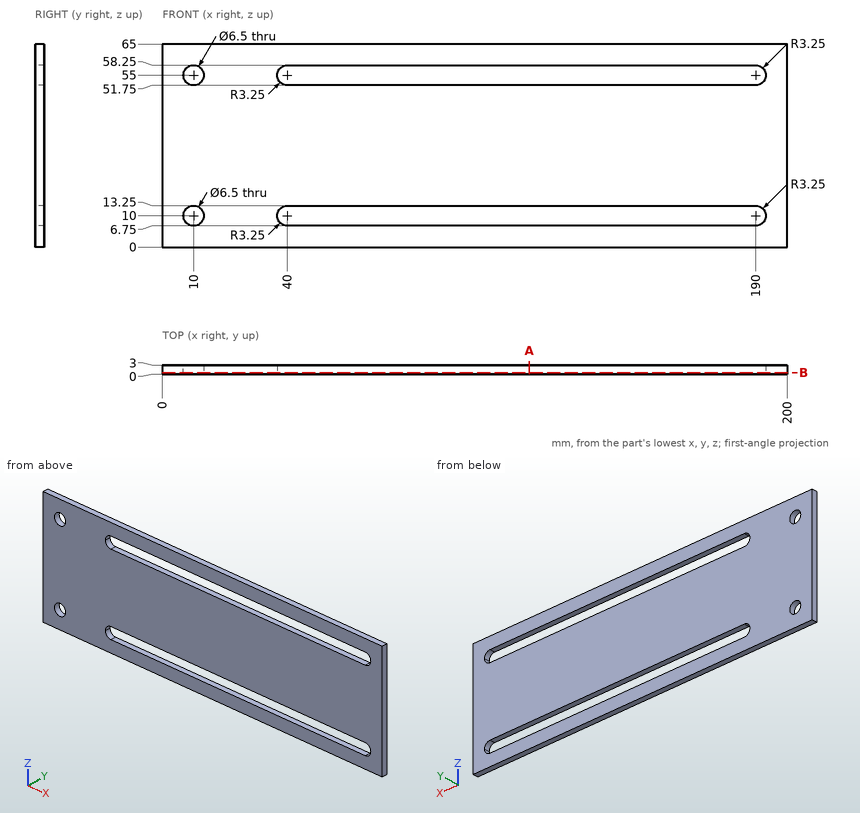
Here's the drawing with two shaded views (mm, measured from the low corner). I have some questions. Coordinates: 2 decimals unless noted, no trailing zeros. Order: outer loops, then holes, each group sorted by start corner. A loop starts at its lowest first (then second) coordinate and runs counter-clockwise, first axis right, second up. Notation, with made-up numbers: (77, 53) - (84, 53) arc R35 ccw to (84, 92) - close; hole circle Ø7 at (-20, 78). An arc over 180 degrees is marked (long way). Use CSV: the item, a comma, the result in double quotes. Start each with the question number.
1. Suppose I cut it at B-B on y = 0.6. List the corners of the cut face in (x, z) for me.
2. Please list where these lines run through material, in increasing order: line 1 (X direction, y = 1.35, z = 10); line 2 (Z direction, x = 87.5, y = 2.4). Write a range as from..to.
3. Suppose I cut it at A-A on x = 117.5. List the corners of the cut face in (y, z) for me, then the cut area to 3 significant figures.
Output:
1,outline,"(0, 0) - (200, 0) - (200, 65) - (0, 65) - close; hole circle Ø6.5 at (10, 10); hole circle Ø6.5 at (10, 55); hole (40, 6.75) - (190, 6.75) arc R3.25 ccw to (190, 13.25) - (40, 13.25) arc R3.25 ccw to start; hole (40, 51.75) - (190, 51.75) arc R3.25 ccw to (190, 58.25) - (40, 58.25) arc R3.25 ccw to start"
2,line 1,"x = 0..6.75, 13.25..36.75, 193.25..200"
2,line 2,"z = 0..6.75, 13.25..51.75, 58.25..65"
3,outline,"(0, 0) - (3, 0) - (3, 6.75) - (0, 6.75) - close; (0, 13.25) - (3, 13.25) - (3, 51.75) - (0, 51.75) - close; (0, 58.25) - (3, 58.25) - (3, 65) - (0, 65) - close"
3,area,"156 mm2"
